Input: dimensioned drawing with shaded views. Units: mm. Origin: part minimum x, y, z. Give positions to 0.01 mm unless a question says otherwise; leave off trailing zeros. Order: outer loops, then holes, each group sorted by start corner. A loop starts at its lowest first (then second) coordinate and runs counter-clockwise, first axis right, second up. Notation, with made-up numbers: M 44.5,78 L 94.5,78 A21 cw 94.5,85 Z; hole C 3,34.5 d3. An arc over 180 degrees is marked long. Answer in a Markdown table with one row per item. Add a question column.
(1) Section query D-D, the plane y = 24.5. Return loops of the section in (x, z), plus the area to 3 significant figures.
(2) Section query B-B, the plane x = 2.54. Return loops of the section in (y, z) (1 decimal), plus the area to 3 significant figures.
(3) Material intervals for line 1 along Z through (x, y) = (56, 50.5), sorted ascending.
(4) Section query A-A, the plane y = 2.54. Return loops of the section in (x, z) (1 decimal).
(5) Section query C-C, the plane z = 10.75. Return loops of the section in (x, y) (1 decimal).
(6) Pin query (flat end, axial travel): P1, Ø8, axis at x = 115, y = 33, coming from the +Z side. Return the tip coordinate at first contact, or that it passes through.
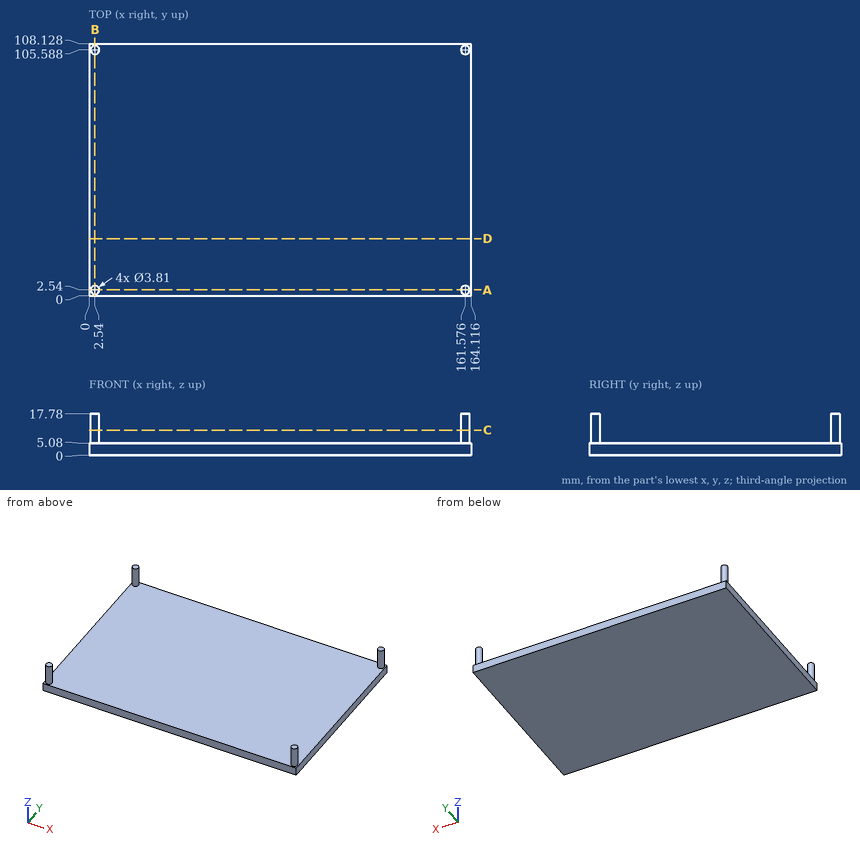
Values follow:
| question | item | result |
|---|---|---|
| 1 | outline | M 0,0 L 164.12,0 L 164.12,5.08 L 0,5.08 Z |
| 1 | area | 834 mm² |
| 2 | outline | M 0,0 L 108.1,0 L 108.1,5.1 L 107.5,5.1 L 107.5,17.8 L 103.7,17.8 L 103.7,5.1 L 4.4,5.1 L 4.4,17.8 L 0.6,17.8 L 0.6,5.1 L 0,5.1 Z |
| 2 | area | 646 mm² |
| 3 | line 1 | z = 0 to 5.08 |
| 4 | outline | M 0,0 L 164.1,0 L 164.1,5.1 L 163.5,5.1 L 163.5,17.8 L 159.7,17.8 L 159.7,5.1 L 4.4,5.1 L 4.4,17.8 L 0.6,17.8 L 0.6,5.1 L 0,5.1 Z |
| 5 | outline | C 2.5,2.5 d3.8; C 2.5,105.6 d3.8; C 161.6,2.5 d3.8; C 161.6,105.6 d3.8 |
| 6 | P1 | stops at z = 5.08 |
